Could you check a few things on this model? Use its own coordinates, in mm. A direction names the side the tool comes from. Coordinates: 2 decimals unless noted, no trailing zeros. Loops run counter-clockwise (first coordinate to the right, second up) from the corner with the lowest first, then second, coordinate; pieces in that order, holes last. Notation, with made-up numbers: (28, -19.75) -> (38, -19.75) arc R30 cw to (38, 19.25) -> close; hole circle Ø1 at (19, 8). An arc over 180 degrees is marked (long way). One line per question, with ' | ' between items. Start each with the question number.
(1) Suppose I cut it at A-A (x = 12). Please give me the cut outline in (y, z).
(2) If I drill on line 1 along Z through (x, y) = (6, 0); line 2 along Y through (x, z) = (1, -0.3); line 3 along Y through (x, z) = (1, -0.05), over which ranges is the centre line in solid material (lowest first)?
(3) Which directions (+Z, -Z, +X, -X, +Y, -Y) give clear straight access to the entire face, cutting with the end or side of a thin tool? Please do faces 1 (the face through (0.15, -1.9, 0.08)), 2 (the face through (9, 0, -1)).
```python
from build123d import *

# Parameters (mm, degrees)
SKETCH3_W         = 0.53
SKETCH3_H         = 2.14
SKETCH4_W         = 0.265
SKETCH4_H         = 0.265
CIRPATTERN1_COUNT = 2
CIRPATTERN1_ANGLE = 90


with BuildPart() as part:
    # BodySke → Base-Revolve (revolve)
    with BuildSketch(Plane.XY):
        Polygon((0, 0), (0, 1.9), (0.3, 1.9), (1.2, 1), (16, 1), (16, 0), align=None)
    revolve(axis=Axis((-6.35, 0, 0), (1, 0, 0)))

    # Sketch3 → Cross section 0
    with BuildSketch(Plane.ZY):
        Rectangle(SKETCH3_W, SKETCH3_H)
    # Sketch4 → Cross section 1
    with BuildSketch(Plane.ZY.offset(-1.54)):
        Rectangle(SKETCH4_W, SKETCH4_H)
    cross = loft(mode=Mode.SUBTRACT)

    # CirPattern1: Cross ×2 about axis
    cirpattern1_axis = Axis((0, 0, 0), (1, 0, 0))
    for i in range(1, CIRPATTERN1_COUNT):
        add(cross.rotate(cirpattern1_axis, i * CIRPATTERN1_ANGLE / (CIRPATTERN1_COUNT - 1)), mode=Mode.SUBTRACT)


solid = part.part
```
Checks:
1) outline: circle Ø2 at (0, 0)
2) line 1: z = -1 to 1 | line 2: y = -1.16 to -0.18, 0.18 to 1.16 | line 3: y = -1.2 to -0.46, 0.46 to 1.2
3) face 1: +X, -X | face 2: +X
